Input: part model. Units: mm. Frame: model coordinates. Face numbers are marked on the shaded views. Give positions to 0.01 mm unless a question says otherwise; leave off trailing zeros. Write each loop counter-clockwise with the first axis right and the second up, starting at its lowest first coordinate (ties: lowest second). Pieces come first, ordered by that corner, then holes. Notation, with made-up numbers: (-3.75, 51) -> (51.25, 51) arc R31 cw to (51.25, 85) -> close; hole circle Ø1 at (76.25, 73). An arc over 180 degrees is marked (long way). Return JSON: item names as keys, results as strings. Group by question number.
Item 1: Section A-A, the plane z = 0. Return loops of the section in (x, y), then the cut area to 3 significant figures.
Item 2: Section B-B, the plane y = -3.5. Return loops of the section in (x, z).
Item 3: Section C-C, the plane x = 16. Return loops of the section in (y, z), then the cut area to 3 significant figures.
Item 4: Mould query, pull axis X, two halves, no side actions, for the marked faces 1, 2 and 3. Classes: released by +X, released by -X, zero draft, split by the parting line, or undercut.
Item 5: Line query: line 1 (Z direction, x = 0, y = -5.5); line 2 (X direction, y = -5.75, z = 0); line 3 (X direction, y = -4, z = 1). Output: solid intervals per line, ascending. Write a range as [from, to].
Item 6: Section D-D, the plane x = 0. Return loops of the section in (y, z).
Item 7: Pin query (flat end, axial travel): P1, Ø4, axis at x = 15, y = -1.5, coming from the -Z side; P2, Ø4, axis at x = 0.5, z = 2, coming from the -Y side. Return the tip coordinate at first contact, or that it passes through.
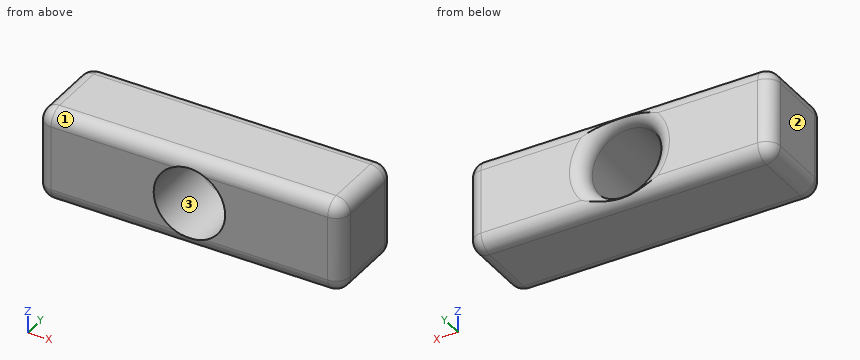
from build123d import *

# Parameters (mm, degrees)
F0_W         = 42.6834902611
F0_H         = 13
F0_R         = 5
F1_DEPTH     = 12
F2_T1_DEPTH  = 8
F2_T3_DEPTH  = 9
F2_T5_DEPTH  = 38.6834902611
F2_S9_W      = 2
F2_S9_H      = 2
F2_T10_DEPTH = 2
F2_S15_W     = 2
F2_S15_H     = 2
F2_T16_DEPTH = 2
F2_S21_W     = 2
F2_S21_H     = 2
F2_T22_DEPTH = 2
F2_S27_W     = 2
F2_S27_H     = 2
F2_T28_DEPTH = 2
F2_S33_W     = 2
F2_S33_H     = 2
F2_T34_DEPTH = 2
F2_S39_W     = 2
F2_S39_H     = 2
F2_T40_DEPTH = 2
F2_S45_W     = 2
F2_S45_H     = 2
F2_T46_DEPTH = 2
F2_S51_W     = 2
F2_S51_H     = 2
F2_T52_DEPTH = 2


# Not quite as in the source:
# - a fillet or chamfer that OpenCascade refuses, or shapes differently, is made with other operations: its cross-section is extruded or revolved along the edge and cut away or added


with BuildPart() as f1:
    # F0 (on Front) → F1 (new body)
    with BuildSketch(Plane.XZ):
        Rectangle(F0_W, F0_H)
        Circle(F0_R, mode=Mode.SUBTRACT)
    extrude(amount=F1_DEPTH)

    # F2: fillet of radius 2 on 13 edges, made by hand

    # F2_s2 → F2_t1 (cut)
    with BuildSketch(Plane.XZ.offset(2)):
        with BuildLine():
            ThreePointArc((-19.3417451306, 6.5), (-20.7559586929, 5.9142135624), (-21.3417451306, 4.5))
            Line((-21.3417451306, 4.5), (-21.3417451306, 6.5))
            Line((-21.3417451306, 6.5), (-19.3417451306, 6.5))
        make_face()
        with BuildLine():
            ThreePointArc((19.3417451306, 6.5), (20.7559586929, 5.9142135624), (21.3417451306, 4.5))
            Line((21.3417451306, 4.5), (21.3417451306, 6.5))
            Line((21.3417451306, 6.5), (19.3417451306, 6.5))
        make_face()
        with BuildLine():
            ThreePointArc((19.3417451306, -6.5), (20.7559586929, -5.9142135624), (21.3417451306, -4.5))
            Line((21.3417451306, -4.5), (21.3417451306, -6.5))
            Line((21.3417451306, -6.5), (19.3417451306, -6.5))
        make_face()
        with BuildLine():
            ThreePointArc((-21.3417451306, -4.5), (-20.7559586929, -5.9142135624), (-19.3417451306, -6.5))
            Line((-19.3417451306, -6.5), (-21.3417451306, -6.5))
            Line((-21.3417451306, -6.5), (-21.3417451306, -4.5))
        make_face()
    extrude(amount=F2_T1_DEPTH, mode=Mode.SUBTRACT)

    # F2_s4 → F2_t3 (cut)
    with BuildSketch(Plane.XY.offset(-4.5)):
        with BuildLine():
            ThreePointArc((21.3417451306, -10), (20.7559586929, -11.4142135624), (19.3417451306, -12))
            Line((19.3417451306, -12), (21.3417451306, -12))
            Line((21.3417451306, -12), (21.3417451306, -10))
        make_face()
        with BuildLine():
            ThreePointArc((21.3417451306, -2), (20.7559586929, -0.5857864376), (19.3417451306, 0))
            Line((19.3417451306, 0), (21.3417451306, 0))
            Line((21.3417451306, 0), (21.3417451306, -2))
        make_face()
        with BuildLine():
            ThreePointArc((-21.3417451306, -10), (-20.7559586929, -11.4142135624), (-19.3417451306, -12))
            Line((-19.3417451306, -12), (-21.3417451306, -12))
            Line((-21.3417451306, -12), (-21.3417451306, -10))
        make_face()
        with BuildLine():
            ThreePointArc((-21.3417451306, -2), (-20.7559586929, -0.5857864376), (-19.3417451306, 0))
            Line((-19.3417451306, 0), (-21.3417451306, 0))
            Line((-21.3417451306, 0), (-21.3417451306, -2))
        make_face()
    extrude(amount=F2_T3_DEPTH, mode=Mode.SUBTRACT)

    # F2_s6 → F2_t5 (cut)
    with BuildSketch(Plane.YZ.offset(-19.3417451306)):
        with BuildLine():
            ThreePointArc((-2, 6.5), (-0.5857864376, 5.9142135624), (0, 4.5))
            Line((0, 4.5), (0, 6.5))
            Line((0, 6.5), (-2, 6.5))
        make_face()
        with BuildLine():
            ThreePointArc((-10, 6.5), (-11.4142135624, 5.9142135624), (-12, 4.5))
            Line((-12, 4.5), (-12, 6.5))
            Line((-12, 6.5), (-10, 6.5))
        make_face()
        with BuildLine():
            ThreePointArc((-2, -6.5), (-0.5857864376, -5.9142135624), (0, -4.5))
            Line((0, -4.5), (0, -6.5))
            Line((0, -6.5), (-2, -6.5))
        make_face()
        with BuildLine():
            ThreePointArc((-10, -6.5), (-11.4142135624, -5.9142135624), (-12, -4.5))
            Line((-12, -4.5), (-12, -6.5))
            Line((-12, -6.5), (-10, -6.5))
        make_face()
    extrude(amount=F2_T5_DEPTH, mode=Mode.SUBTRACT)


with BuildPart() as f2_tool8:
    # F2_s9 → F2_t10 (new body)
    with BuildSketch(Plane.XY.offset(4.5)):
        with Locations((-20.3417451306, -1)):
            Rectangle(F2_S9_W, F2_S9_H)
    extrude(amount=F2_T10_DEPTH)

    # F2_s11 → F2_t12 (revolve, cut)
    with BuildSketch(Plane(origin=(-19.3417451306, -2, 4.5), x_dir=(0.7071067812, -0.7071067812, 0), z_dir=(-0.7071067812, -0.7071067812, 0))):
        with BuildLine():
            ThreePointArc((0, -2), (2, 0), (0, 2))
            Line((0, 2), (0, -2))
        make_face()
    revolve(axis=Axis((-19.3417451306, -2, 4.5), (0, 0, 1)), mode=Mode.SUBTRACT)


with BuildPart() as f1_1:
    add(f1.part)

    # F2_t7: cut F2_tool8
    add(f2_tool8.part, mode=Mode.SUBTRACT)


with BuildPart() as f2_tool14:
    # F2_s15 → F2_t16 (new body)
    with BuildSketch(Plane.XY.offset(4.5)):
        with Locations((-20.3417451306, -11)):
            Rectangle(F2_S15_W, F2_S15_H)
    extrude(amount=F2_T16_DEPTH)

    # F2_s17 → F2_t18 (revolve, cut)
    with BuildSketch(Plane(origin=(-19.3417451306, -10, 4.5), x_dir=(0.7071067812, 0.7071067812, 0), z_dir=(0.7071067812, -0.7071067812, 0))):
        with BuildLine():
            ThreePointArc((0, -2), (2, 0), (0, 2))
            Line((0, 2), (0, -2))
        make_face()
    revolve(axis=Axis((-19.3417451306, -10, 4.5), (0, 0, 1)), mode=Mode.SUBTRACT)


with BuildPart() as f1_2:
    add(f1_1.part)

    # F2_t13: cut F2_tool14
    add(f2_tool14.part, mode=Mode.SUBTRACT)


with BuildPart() as f2_tool20:
    # F2_s21 → F2_t22 (new body)
    with BuildSketch(Plane.XY.offset(4.5)):
        with Locations((20.3417451306, -1)):
            Rectangle(F2_S21_W, F2_S21_H)
    extrude(amount=F2_T22_DEPTH)

    # F2_s23 → F2_t24 (revolve, cut)
    with BuildSketch(Plane(origin=(19.3417451306, -2, 4.5), x_dir=(-0.7071067812, -0.7071067812, 0), z_dir=(-0.7071067812, 0.7071067812, 0))):
        with BuildLine():
            ThreePointArc((0, -2), (2, 0), (0, 2))
            Line((0, 2), (0, -2))
        make_face()
    revolve(axis=Axis((19.3417451306, -2, 4.5), (0, 0, 1)), mode=Mode.SUBTRACT)


with BuildPart() as f1_3:
    add(f1_2.part)

    # F2_t19: cut F2_tool20
    add(f2_tool20.part, mode=Mode.SUBTRACT)


with BuildPart() as f2_tool26:
    # F2_s27 → F2_t28 (new body)
    with BuildSketch(Plane.XY.offset(4.5)):
        with Locations((20.3417451306, -11)):
            Rectangle(F2_S27_W, F2_S27_H)
    extrude(amount=F2_T28_DEPTH)

    # F2_s29 → F2_t30 (revolve, cut)
    with BuildSketch(Plane(origin=(19.3417451306, -10, 4.5), x_dir=(-0.7071067812, 0.7071067812, 0), z_dir=(0.7071067812, 0.7071067812, 0))):
        with BuildLine():
            ThreePointArc((0, -2), (2, 0), (0, 2))
            Line((0, 2), (0, -2))
        make_face()
    revolve(axis=Axis((19.3417451306, -10, 4.5), (0, 0, 1)), mode=Mode.SUBTRACT)


with BuildPart() as f1_4:
    add(f1_3.part)

    # F2_t25: cut F2_tool26
    add(f2_tool26.part, mode=Mode.SUBTRACT)


with BuildPart() as f2_tool32:
    # F2_s33 → F2_t34 (new body)
    with BuildSketch(Plane.XY.offset(-4.5)):
        with Locations((20.3417451306, -1)):
            Rectangle(F2_S33_W, F2_S33_H)
    extrude(amount=-F2_T34_DEPTH)

    # F2_s35 → F2_t36 (revolve, cut)
    with BuildSketch(Plane(origin=(19.3417451306, -2, -4.5), x_dir=(-0.7071067812, -0.7071067812, 0), z_dir=(0.7071067812, -0.7071067812, 0))):
        with BuildLine():
            ThreePointArc((0, -2), (2, 0), (0, 2))
            Line((0, 2), (0, -2))
        make_face()
    revolve(axis=Axis((19.3417451306, -2, -4.5), (0, 0, -1)), mode=Mode.SUBTRACT)


with BuildPart() as f1_5:
    add(f1_4.part)

    # F2_t31: cut F2_tool32
    add(f2_tool32.part, mode=Mode.SUBTRACT)


with BuildPart() as f2_tool38:
    # F2_s39 → F2_t40 (new body)
    with BuildSketch(Plane.XY.offset(-4.5)):
        with Locations((20.3417451306, -11)):
            Rectangle(F2_S39_W, F2_S39_H)
    extrude(amount=-F2_T40_DEPTH)

    # F2_s41 → F2_t42 (revolve, cut)
    with BuildSketch(Plane(origin=(19.3417451306, -10, -4.5), x_dir=(-0.7071067812, 0.7071067812, 0), z_dir=(-0.7071067812, -0.7071067812, 0))):
        with BuildLine():
            ThreePointArc((0, -2), (2, 0), (0, 2))
            Line((0, 2), (0, -2))
        make_face()
    revolve(axis=Axis((19.3417451306, -10, -4.5), (0, 0, -1)), mode=Mode.SUBTRACT)


with BuildPart() as f1_6:
    add(f1_5.part)

    # F2_t37: cut F2_tool38
    add(f2_tool38.part, mode=Mode.SUBTRACT)


with BuildPart() as f2_tool44:
    # F2_s45 → F2_t46 (new body)
    with BuildSketch(Plane.YZ.offset(-19.3417451306)):
        with Locations((-11, -5.5)):
            Rectangle(F2_S45_W, F2_S45_H)
    extrude(amount=-F2_T46_DEPTH)

    # F2_s47 → F2_t48 (revolve, cut)
    with BuildSketch(Plane(origin=(-19.3417451306, -10, -4.5), x_dir=(0, 0.7071067812, 0.7071067812), z_dir=(0, -0.7071067812, 0.7071067812))):
        with BuildLine():
            ThreePointArc((0, -2), (2, 0), (0, 2))
            Line((0, 2), (0, -2))
        make_face()
    revolve(axis=Axis((-19.3417451306, -10, -4.5), (-1, 0, 0)), mode=Mode.SUBTRACT)


with BuildPart() as f1_7:
    add(f1_6.part)

    # F2_t43: cut F2_tool44
    add(f2_tool44.part, mode=Mode.SUBTRACT)


with BuildPart() as f2_tool50:
    # F2_s51 → F2_t52 (new body)
    with BuildSketch(Plane.YZ.offset(-19.3417451306)):
        with Locations((-1, -5.5)):
            Rectangle(F2_S51_W, F2_S51_H)
    extrude(amount=-F2_T52_DEPTH)

    # F2_s53 → F2_t54 (revolve, cut)
    with BuildSketch(Plane(origin=(-19.3417451306, -2, -4.5), x_dir=(0, -0.7071067812, 0.7071067812), z_dir=(0, -0.7071067812, -0.7071067812))):
        with BuildLine():
            ThreePointArc((0, -2), (2, 0), (0, 2))
            Line((0, 2), (0, -2))
        make_face()
    revolve(axis=Axis((-19.3417451306, -2, -4.5), (-1, 0, 0)), mode=Mode.SUBTRACT)


with BuildPart() as f1_8:
    add(f1_7.part)

    # F2_t49: cut F2_tool50
    add(f2_tool50.part, mode=Mode.SUBTRACT)

    # F2_s55 → F2_t56 (revolve, cut)
    with BuildSketch(Plane.XY):
        with BuildLine():
            ThreePointArc((5, -2), (5.5857864376, -0.5857864376), (7, 0))
            Line((7, 0), (5, 0))
            Line((5, 0), (5, -2))
        make_face()
    revolve(axis=Axis((0, 0, 0), (0, -1, 0)), mode=Mode.SUBTRACT)


solid = f1_8.part
Answer below:
{
 "1": {"outline": "(-21.34, -10) arc R2 ccw to (-19.34, -12) -> (-5, -12) -> (-5, -2) arc R2 ccw to (-7, 0) -> (-19.34, 0) arc R2 ccw to (-21.34, -2) -> close; (5, -12) -> (19.34, -12) arc R2 ccw to (21.34, -10) -> (21.34, -2) arc R2 ccw to (19.34, 0) -> (7, 0) arc R2 ccw to (5, -2) -> close", "area": "387 mm2"},
 "2": {"outline": "(-21.34, -4.5) arc R2 ccw to (-19.34, -6.5) -> (19.34, -6.5) arc R2 ccw to (21.34, -4.5) -> (21.34, 4.5) arc R2 ccw to (19.34, 6.5) -> (-19.34, 6.5) arc R2 ccw to (-21.34, 4.5) -> close; hole circle Ø10 at (0, 0)"},
 "3": {"outline": "(-12, -4.5) arc R2 ccw to (-10, -6.5) -> (-2, -6.5) arc R2 ccw to (0, -4.5) -> (0, 4.5) arc R2 ccw to (-2, 6.5) -> (-10, 6.5) arc R2 ccw to (-12, 4.5) -> close", "area": "153 mm2"},
 "4": {"face 1": "zero draft", "face 2": "released by -X", "face 3": "undercut"},
 "5": {"line 1": "z = [-6.5, -5], [5, 6.5]", "line 2": "x = [-21.34, -5], [5, 21.34]", "line 3": "x = [-21.34, -4.9], [4.9, 21.34]"},
 "6": {"outline": "(-11.94, -5) arc R2 ccw to (-10, -6.5) -> (-2, -6.5) arc R2 ccw to (-0.44, -5.75) arc R2 ccw to (-2, -5) -> close; (-11.94, 5) -> (-2, 5) arc R2 ccw to (-0.44, 5.75) arc R2 ccw to (-2, 6.5) -> (-10, 6.5) arc R2 ccw to start"},
 "7": {"P1": "stops at z = -6.5", "P2": "passes through"}
}
